```python
from build123d import *

# Parameters (mm, degrees)
ESBO_O1_W                = 19
ESBO_O1_H                = 19
RESSALTO_EXTRUS_O1_DEPTH = 260
CASCA2_T                 = -1
CORTE_EXTRUS_O1_DEPTH    = 261.866345089
CORTE_EXTRUS_O3_DEPTH    = 261.866345089
ESBO_O5_R                = 1.5
CORTE_EXTRUS_O4_DEPTH    = 170.569790677


with BuildPart() as part:
    # Esboço1 → Ressalto-extrusão1 (new body)
    with BuildSketch(Plane.XY):
        Rectangle(ESBO_O1_W, ESBO_O1_H)
    extrude(amount=RESSALTO_EXTRUS_O1_DEPTH)

    # Casca2
    casca2_openings = [part.faces().sort_by_distance(p)[0] for p in [
        (0, 0, 260),
        (0, 0, 0),
    ]]
    offset(amount=CASCA2_T, openings=casca2_openings, kind=Kind.INTERSECTION)

    # Esboço2 → Corte-extrusão1 (cut, through all)
    with BuildSketch(Plane(origin=(9.5, 0, 0), x_dir=(0, 0, -1), z_dir=(1, 0, 0))):
        Polygon((0, 9.5), (-58.475987206, -9.5), (0, -9.5), align=None)
    extrude(amount=-CORTE_EXTRUS_O1_DEPTH, mode=Mode.SUBTRACT)

    # Esboço4 → Corte-extrusão3 (cut, through all)
    with BuildSketch(Plane(origin=(9.5, 0, 0), x_dir=(0, 0, -1), z_dir=(1, 0, 0))):
        Polygon((-168.550335734, 10.473717073), (-161.289503816, -11.872825786), (-264.812755879, -45.509569399), (-289.05777752, 22.149749677), (-184.516070462, 59.611196004), align=None)
    extrude(amount=-CORTE_EXTRUS_O3_DEPTH, mode=Mode.SUBTRACT)

    # Esboço5 → Corte-extrusão4 (cut, through all)
    with BuildSketch(Plane(origin=(0, 9.5, 0), x_dir=(1, 0, 0), z_dir=(0, 1, 0))):
        with Locations(Location((0, -20, 0), (0, 0, 270))):
            Circle(ESBO_O5_R)
        with Locations(Location((0, -45, 0), (0, 0, 270))):
            Circle(ESBO_O5_R)
    extrude(amount=-CORTE_EXTRUS_O4_DEPTH, mode=Mode.SUBTRACT)


solid = part.part
```
Read the model definition and answer for the solid it produces. Units are mm, in the model's axes. A direction names the side the tool comes from. Give positions to 0.01 mm unless a question says otherwise; leave off trailing zeros. Write each loop counter-clockwise with the first axis right and the second up, starting at its lowest first coordinate (ties: lowest second). Pieces come first, ordered by that corner, then holes. Notation, with made-up numbers: (-6, -34.75) - (29, -34.75) arc R30 ccw to (29, -6.75) - close; hole circle Ø9 at (-24.75, 46). An arc over 180 degrees is marked (long way). Write item = value, one per line. Start each with the question number.
Item 1: Find the intervals of material crossed by probe 1 along X at (y, z) = (3.5, 143.5); probe 2 along X at (y, z) = (9.15, 20), in increasing order. Write a range as [from, to].
Item 2: Find section C-C (z = 45). Give the vertices of the cut face in (x, y).
Item 3: A tool of negligible diameter and unlimited length cuts with its end or side. For faces 5 (the flat face through (9.5, 0, 102)), 6 (the flat face through (-8.5, 0, 103)), from which of +Z, -Z, +X, -X, +Y, -Y can it reach the whole face along a straight path? Write none if from no direction.
Item 4: Find section B-B (y = -5.5). Give the vertices of the cut face in (x, z), then the cut area to 3 significant figures.
Item 5: The mould has two halves that part along X. Classify faces 1 (the flat face through (-9.5, 0, 102)), 2 (the flat face through (-9.1, 0.75, 165.39)), 3 (the flat face through (0, -8.5, 108)), 4 (the flat face through (0, 8.5, 84)): +X half, -X half, draft (parallel to the pull), parting line (faces both ways), or undercut.
Item 6: Find section D-D (z = 63). Give the vertices of the cut face in (x, y), then the cut area to 3 significant figures.
Item 7: Find section A-A (x = 0). Give the vertices of the cut face in (y, z).
Response:
q1.probe_1 = [-9.5, -8.5], [8.5, 9.5]
q1.probe_2 = [-9.5, -1.5], [1.5, 9.5]
q2.outline = (-9.5, -5.12) - (-8.5, -5.12) - (-8.5, 8.5) - (-1.5, 8.5) - (-1.5, 9.5) - (-9.5, 9.5) - close; (1.5, 8.5) - (8.5, 8.5) - (8.5, -5.12) - (9.5, -5.12) - (9.5, 9.5) - (1.5, 9.5) - close
q3.face_5 = +Z, -Z, +X, +Y, -Y
q3.face_6 = +Z, -Z
q4.outline = (-9.5, 46.17) - (-8.5, 46.17) - (-8.5, 163.36) - (-9.5, 163.36) - close; (8.5, 46.17) - (9.5, 46.17) - (9.5, 163.36) - (8.5, 163.36) - close
q4.area = 234 mm²
q5.face_1 = -X half
q5.face_2 = draft
q5.face_3 = undercut
q5.face_4 = undercut
q6.outline = (-9.5, -9.5) - (9.5, -9.5) - (9.5, 9.5) - (-9.5, 9.5) - close; hole (-8.5, -8.5) - (8.5, -8.5) - (8.5, 8.5) - (-8.5, 8.5) - close
q6.area = 72.0 mm²
q7.outline = (-9.5, 58.48) - (-8.5, 55.4) - (-8.5, 162.39) - (-9.5, 162.06) - close; (8.5, 3.08) - (9.5, 0) - (9.5, 18.5) - (8.5, 18.5) - close; (8.5, 21.5) - (9.5, 21.5) - (9.5, 43.5) - (8.5, 43.5) - close; (8.5, 46.5) - (9.5, 46.5) - (9.5, 168.23) - (8.5, 167.91) - close
